Can you work these out from the drawing? Everything is in mm from the part's minimum corner. A direction names the side the tool comes from. Round coordinates to 2 decimals unless told otherwise and drop trailing zeros. Write each loop counter-clockwise with the first axis right and the second up, starting at its lowest first coordinate (ties: lowest second). Pieces come first, ordered by that corner, then holes.
Q1. For the marked faces 1, 2 and 3, which set-ups out of +Z, -Z, +X, -X, +Y, -Y let a thin tool reach every point of the face, with its end or its side?
Q2. We'd pull the mould along Z, two halves only. Please class the marked faces 4, 5 and 6: +Z half, -Z half, draft (parallel to the pull), parting line (faces both ways), or undercut.
Q3. If we section it at B-B (z = 64.5): Please give me the cut outline in (x, y), plus the area to 3 significant figures.
Q4. Please list where these lines run through material, in increasing order: line 1 along X through (y, z) = (20.5, 57.5); line 2 along X through (y, z) = (18.5, 67); line 3 along Z through (x, y) = (26.5, 5.75).
Q5. If we section it at A-A (y = 15.5): Please give me the cut outline in (x, z), plus the area to 3 significant figures.
Q6. If we section it at C-C (x = 35): Please give me the cut outline in (y, z).
Q7. If we section it at D-D (y = 21): Please give me the cut outline in (x, z).
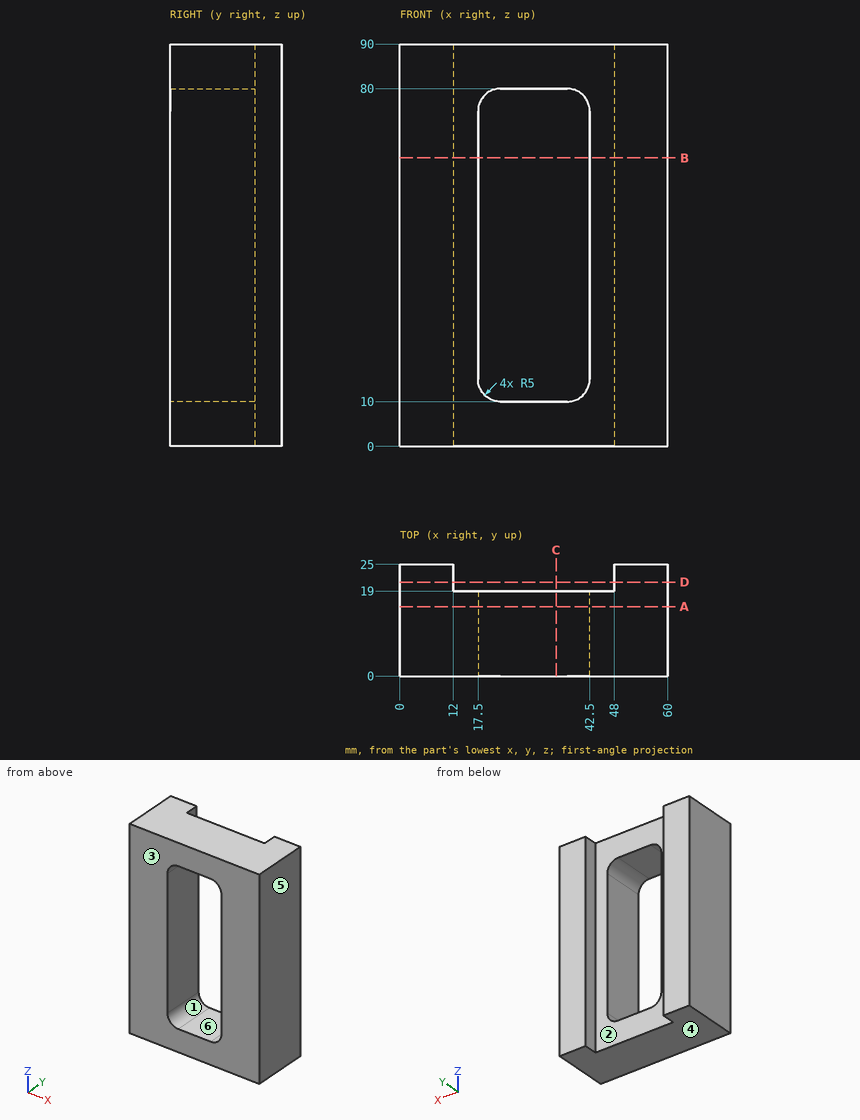
A:
1. face 1: +Y, -Y
1. face 2: +Z, -Z, +Y
1. face 3: +Z, -Z, +X, -X, -Y
2. face 4: -Z half
2. face 5: draft
2. face 6: undercut
3. outline: (0, 0) - (17.5, 0) - (17.5, 19) - (12, 19) - (12, 25) - (0, 25) - close; (42.5, 0) - (60, 0) - (60, 25) - (48, 25) - (48, 19) - (42.5, 19) - close
3. area: 809 mm2
4. line 1: x = 0 to 12, 48 to 60
4. line 2: x = 0 to 17.5, 42.5 to 60
4. line 3: z = 0 to 10, 80 to 90
5. outline: (0, 0) - (60, 0) - (60, 90) - (0, 90) - close; hole (17.5, 15) arc R5 ccw to (22.5, 10) - (37.5, 10) arc R5 ccw to (42.5, 15) - (42.5, 75) arc R5 ccw to (37.5, 80) - (22.5, 80) arc R5 ccw to (17.5, 75) - close
5. area: 3,670 mm2
6. outline: (0, 0) - (19, 0) - (19, 10) - (0, 10) - close; (0, 80) - (19, 80) - (19, 90) - (0, 90) - close
7. outline: (0, 0) - (12, 0) - (12, 90) - (0, 90) - close; (48, 0) - (60, 0) - (60, 90) - (48, 90) - close
